Source: CAD feature listing. Evaluate the final solid. Frame: model axes, mm. A direction names the side the tool comes from. Give positions to 0.01 mm unless a question says otherwise; leave off trailing zeros. Order: outer loops, then holes, each group sorted by start corner. A loop starts at its lowest first (then second) coordinate and runs counter-clockwise, first axis right, second up. Notation, with made-up numbers: M 72,40 L 82,40 A21 cw 82,74 Z; hole C 50,64 d1. An arc over 180 degrees is marked long. Answer in a Markdown table with one row per item. Add a question column.
(1) Section query A-A, the plane y = -38.1. Return loops of the section in (x, z), plus the area to 3 significant figures.
(2) Set-up query: faces 1 (the face through (0, 0, -7)), 2 (the face through (25.4, 1, 17)). Return all of +Z, -Z, +X, -X, +Y, -Y with unobstructed straight access to the full face (end or side cutting, diameter ignored); none if empty.
(3) Section query B-B, the plane x = 0. Return loops of the section in (y, z), plus the area to 3 significant figures.
(4) Pin query (flat end, axial travel): P1, Ø9.5, axis at x = 0, y = -38.1, coming from the -Z side; P2, Ø10, axis at x = 19.5, z = 1.5, coming from the +Y side; P3, Ø8, axis at x = 1, y = -2.5, coming from the -Z side. Return the tip coordinate at first contact, or that it passes through.
(5) Material intervals for line 1 along X through (y, z) = (-38.1, 32.5); line 2 along Y through (x, z) = (0, 29); line 3 along Z through (x, y) = (19, -34), sorted ascending.
(6) Mould query, pull axis X, two halves, no side actions, for faces 3 (the face through (3.86, 50.27, 5.04)), 4 (the face through (-0.672, -32.985, 32.099)), 5 (the face through (0, 88.9, 0)). Classes: pulls with the +X half, pulls with the -X half, needs draft (parallel to the pull), parting line crosses it, or undercut.
(7) Section query D-D, the plane z = 0. Return loops of the section in (x, y).
(8) Section query C-C, the plane z = 32.5. Return loops of the section in (x, y), plus the area to 3 significant figures.
from build123d import *

# Parameters (mm, degrees)
SKETCH1_W                                  = 50.8
SKETCH1_H                                  = 76.2
BOSS_EXTRUDE1_DEPTH                        = 12.7
SKETCH2_R                                  = 6.35
BOSS_EXTRUDE2_DEPTH                        = 76.2
SKETCH4_W                                  = 50.8
SKETCH4_H                                  = 12.808038323
BOSS_EXTRUDE3_DEPTH                        = 76.2
F_13_32_0_40625_DIAMETER_HOLE1_D           = 10.31875
F_13_32_0_40625_DIAMETER_HOLE1_CSINK_D     = 11.58875
F_13_32_0_40625_DIAMETER_HOLE1_CSINK_ANGLE = 90


with BuildPart() as part:
    # Sketch1 → Boss-Extrude1 (new body)
    with BuildSketch(Plane(origin=(0, 0, 0), x_dir=(1, 0, 0), z_dir=(0, 1, 0))):
        Rectangle(SKETCH1_W, SKETCH1_H)
    extrude(amount=BOSS_EXTRUDE1_DEPTH)

    # Sketch2 → Boss-Extrude2 (add)
    with BuildSketch(Plane(origin=(0, 12.7, 0), x_dir=(1, 0, 0), z_dir=(0, 1, 0))):
        with Locations(Location((0, 0, 0), (0, 0, 90))):
            Circle(SKETCH2_R)
    extrude(amount=BOSS_EXTRUDE2_DEPTH)

    # Sketch4 → Boss-Extrude3 (add)
    with BuildSketch(Plane(origin=(0, 12.7, 0), x_dir=(1, 0, 0), z_dir=(0, 1, 0))):
        with Locations((0, -31.695980839)):
            Rectangle(SKETCH4_W, SKETCH4_H)
    extrude(amount=-BOSS_EXTRUDE3_DEPTH)

    # 13/32 (0.40625) Diameter Hole1 (through all)
    with Locations(Plane(origin=(0, 0, 25.291961677), x_dir=(-1, 0, 0), z_dir=(0, 0, -1))):
        with Locations((0, -38.1)):
            CounterSinkHole(F_13_32_0_40625_DIAMETER_HOLE1_D / 2, F_13_32_0_40625_DIAMETER_HOLE1_CSINK_D / 2, counter_sink_angle=F_13_32_0_40625_DIAMETER_HOLE1_CSINK_ANGLE)


solid = part.part
Values follow:
| question | item | result |
|---|---|---|
| 1 | outline | M -25.4,25.29 L -5.79,25.29 L -5.16,25.93 L -5.16,38.1 L -25.4,38.1 Z; M 5.16,25.93 L 5.79,25.29 L 25.4,25.29 L 25.4,38.1 L 5.16,38.1 Z |
| 1 | area | 518 mm² |
| 2 | face 1 | -Z, +X, -X, -Y |
| 2 | face 2 | +Z, -Z, +X, +Y, -Y |
| 3 | outline | M -63.5,25.29 L -43.89,25.29 L -43.26,25.93 L -43.26,38.1 L -63.5,38.1 Z; M -32.94,25.93 L -32.31,25.29 L 0,25.29 L 0,-38.1 L 12.7,-38.1 L 12.7,-6.35 L 88.9,-6.35 L 88.9,6.35 L 12.7,6.35 L 12.7,38.1 L -32.94,38.1 Z |
| 3 | area | 2,620 mm² |
| 4 | P1 | passes through |
| 4 | P2 | stops at y = 12.7 |
| 4 | P3 | stops at z = -38.1 |
| 5 | line 1 | x = -25.4 to -5.16, 5.16 to 25.4 |
| 5 | line 2 | y = -63.5 to -43.26, -32.94 to 12.7 |
| 5 | line 3 | z = 25.29 to 38.1 |
| 6 | face 3 | parting line crosses it |
| 6 | face 4 | undercut |
| 6 | face 5 | needs draft |
| 7 | outline | M -25.4,0 L 25.4,0 L 25.4,12.7 L 6.35,12.7 L 6.35,88.9 L -6.35,88.9 L -6.35,12.7 L -25.4,12.7 Z |
| 8 | outline | M -25.4,-63.5 L 25.4,-63.5 L 25.4,12.7 L -25.4,12.7 Z; hole C 0,-38.1 d10.32 |
| 8 | area | 3,790 mm² |
